The model under review builds one solid part; all positions refer to its coordinate system, in mm. Coordinates: 2 decimals unless noted, no trailing zeros. Write each loop counter-clockwise with the first axis right and the second up, starting at its lowest first coordinate (ties: lowest second). Pieces come first, ordered by that corner, then holes. Notation, with made-up numbers: (66.5, 18) -> (91.5, 18) arc R6 ccw to (91.5, 28) -> close; hole circle Ø3 at (-31, -16). An arc over 180 degrees is marked (long way). Put each result on its own line as item: value. Start each with the question number.
from build123d import *

# Parameters (mm, degrees)
SKETCH_1_W          = 40
SKETCH_1_H          = 20
SKETCH_1_W_2        = 38
SKETCH_1_H_2        = 18
EXTRUDE_1_DEPTH     = 670
SKETCH_4_R          = 1.75
CUT_EXTRUDE_2_DEPTH = 1.5
SKETCH_8_R          = 1.65
CUT_EXTRUDE_3_DEPTH = 5


with BuildPart() as part:
    # 草图1 → 拉伸-薄壁1 (new body)
    with BuildSketch(Plane.XY):
        with Locations((20, -10)):
            Rectangle(SKETCH_1_W, SKETCH_1_H)
        with Locations((20, -10)):
            Rectangle(SKETCH_1_W_2, SKETCH_1_H_2, mode=Mode.SUBTRACT)
    extrude(amount=EXTRUDE_1_DEPTH)

    # 草图4 → 切除-拉伸2 (cut)
    with BuildSketch(Plane.ZY):
        with Locations((659.996387591, -10)):
            Circle(SKETCH_4_R)
        with Locations((10, -10.000000002)):
            Circle(SKETCH_4_R)
    extrude(amount=-CUT_EXTRUDE_2_DEPTH, mode=Mode.SUBTRACT)

    # 草图8 → 切除-拉伸3 (cut)
    with BuildSketch(Plane.ZY):
        with Locations((100, -7.5)):
            Circle(SKETCH_8_R)
        with Locations((370, -7.5)):
            Circle(SKETCH_8_R)
    extrude(amount=-CUT_EXTRUDE_3_DEPTH, mode=Mode.SUBTRACT)


solid = part.part
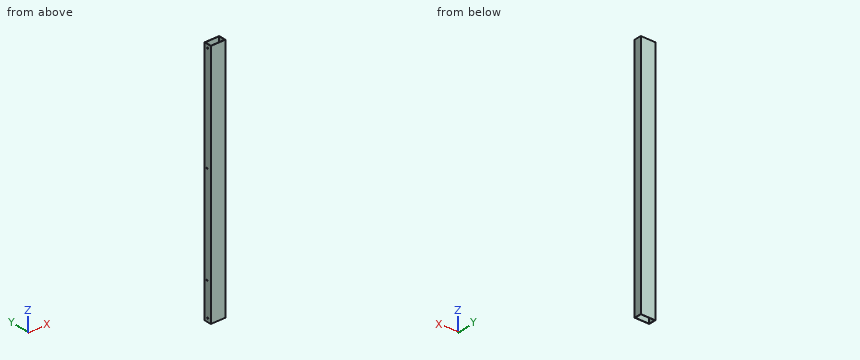
1. Consider section B-B on z = 255. State the section outline as (x, y) points.
2. Consider section A-A on x = 8. State the section outline as (y, z) points.
3. Wall thickness on line 1 (Y direction, x = 0.6, z = 100); line 2 (X direction, y = -2.5, z = 247); line 3 (Y direction, x = 3.5, z = 442.5): over which ranges is each line inside the solid? List them lowest first. Write a range as from..to.
4. Insertion check: P1, Ø3, axis at y = -10, z = 10, coming from the -X side. The pin has a flat end and moves straight along its axis. Give the tip position at first contact, or say it passes through.
Output values:
1. outline: (0, -20) -> (40, -20) -> (40, 0) -> (0, 0) -> close; hole (1, -19) -> (39, -19) -> (39, -1) -> (1, -1) -> close
2. outline: (-20, 0) -> (-19, 0) -> (-19, 670) -> (-20, 670) -> close; (-1, 0) -> (0, 0) -> (0, 670) -> (-1, 670) -> close
3. line 1: y = -20..-9.15, -5.85..0
3. line 2: x = 0..1, 39..40
3. line 3: y = -20..-19, -1..0
4. P1: stops at x = 39
